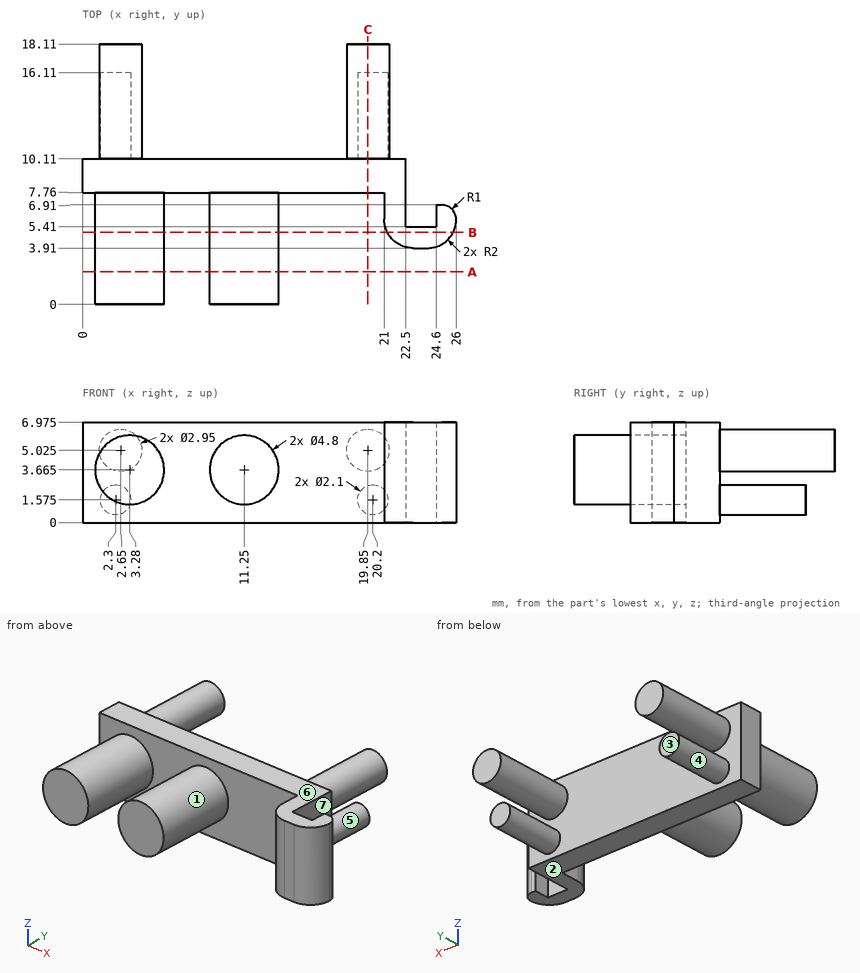
Check sheet for the drawn part. Datum: minimum x, y, z corner. Units: mm. A direction names the side the tool comes from. Coordinates: 2 decimals unless noted, no trailing zeros. Loops run counter-clockwise (first coordinate to the right, second up) from the corner with the lowest first, then second, coordinate; pieces in that order, holes last. Notation, with made-up numbers: M 45,67 L 85,67 A16 ccw 85,92 Z; hole C 58,-35.5 d10. An arc over 180 degrees is marked long. Answer as a JSON object with one key per item and string values.
1. Release check for a two-part mould opening along Z. For the marked faces 5, 6 and 7 record: pulls with the +Z half, pulls with the -Z half, needs draft (parallel to the pull), parting line crosses it, or undercut.
Outcome:
{"face 5": "undercut", "face 6": "pulls with the +Z half", "face 7": "needs draft"}
2. Sectioned sample at B-B on y = 5. Record the cut outline in (x, z) (3 decimals), and give its area (3 significant figures).
Outcome:
{"outline": "C 3.28,3.665 d4.8; C 11.25,3.665 d4.8; M 21.219,0 L 25.781,0 L 25.781,6.975 L 21.219,6.975 Z", "area": "68.0 mm²"}
3. Depth check by flat-ended pin: P1, Ø0.8, axis at x = 23.5, z = 5, coming from the -Y side; P2, Ø1.5, axis at y = 5.5, z = 5, coming from the -X side; P3, Ø1.4, axis at y = 8.5, z = 3, coming from the +X side. Enter the tip coordinate at first touch or a pass-through.
Outcome:
{"P1": "y = 3.91", "P2": "x = 0.95", "P3": "x = 22.5"}
4. Scan lines: L1, parallel to X at y = 4.5, z = 5.25; L2, parallel to Y at x = 23, z = 1; L3, parallel to X at y = 6, z = 5.25. Record each from-to range of solid material in increasing order. Write a range as from..to.
Outcome:
{"L1": "1.48..5.08, 9.45..13.05, 21.58..25.42", "L2": "3.91..5.41", "L3": "1.48..5.08, 9.45..13.05, 21..22.5, 24.6..26"}
5. Sectioned sample at A-A on y = 2.25. Record the cut outline in (x, z) (3 decimals), and give its area (3 significant figures).
Outcome:
{"outline": "C 3.28,3.665 d4.8; C 11.25,3.665 d4.8", "area": "36.2 mm²"}
6. Access from +Z, -Z, +X, -X, +Y, -Y to the whole of each face (thin tool, end or side, straight path). Record for the marked faces 1, 2, 3 and 4.
Outcome:
{"face 1": "-Y", "face 2": "-Z, +X, -X, +Y, -Y", "face 3": "-Z, +X, -X, +Y", "face 4": "+Y"}
7. Sectioned sample at C-C on x = 19.85. Record the cut outline in (y, z) (3 decimals), and give its area (3 significant figures).
Outcome:
{"outline": "M 7.76,0 L 10.11,0 L 10.11,0.585 L 16.11,0.585 L 16.11,2.565 L 10.11,2.565 L 10.11,3.55 L 18.11,3.55 L 18.11,6.5 L 10.11,6.5 L 10.11,6.975 L 7.76,6.975 Z", "area": "51.9 mm²"}
